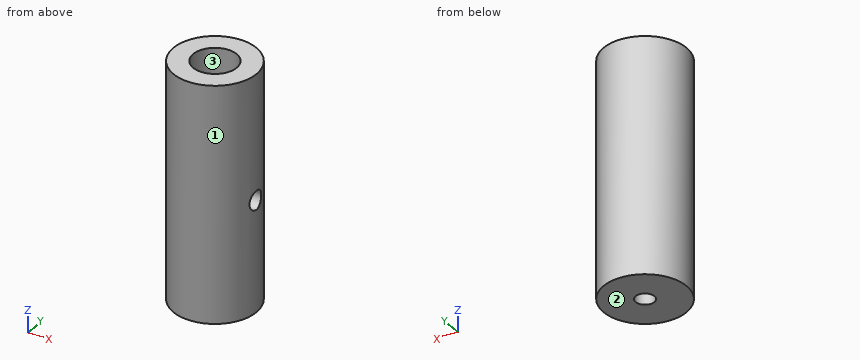
Autodesk Inventor part; units mm, degrees
ref_plane "Work Plane1" through (4.7625, 0, 0) normal (1, 0, 0) x (0, 1, 0)
ref_plane "XZ Plane" through (0, 0, 0) normal (0, 1, 0) x (-1, 0, 0)
ref_plane "XY Plane" through (0, 0, 0) normal (0, 0, 1) x (1, 0, 0)
sketch "Sketch1" plane through (0, 0, 0) normal (0, 0, 1) x (1, 0, 0)
  circle A0 centre (0, 0) radius 4.7625
  dimension "d0" = 9.525
extrude "Extrusion1" add sketch "Sketch1" along normal blind 26.9875
sketch "Sketch2" plane through (0, 0, 26.9875) normal (0, 0, 1) x (1, 0, 0)
  point P0 (0, 0)
  point P1 (0, 0)
hole "Hole1" at (0, 0, 26.9875) direction (0, 0, -1) diameter 5 depth 20.6375 tip angle 118
sketch "Sketch3" plane through (0, 0, 0) normal (0, 0, -1) x (-1, 0, 0)
  circle A0 centre (0, 0) radius 4.7625
hole "Hole2" at (0, 0, 0) direction (0, 0, 1) diameter 2.159 depth 8.8646 tip angle 118
ref_plane "Work Plane1" through (4.7625, 0, 0) normal (1, 0, 0) x (0, 1, 0)
sketch "Sketch4" plane through (4.7625, 0, 0) normal (1, 0, 0) x (0, 1, 0)
  line L0 (-2.5, 26.9875) -> (2.5, 26.9875)
  line L1 (0, 26.9875) -> (0, 12.7)
  point P0 (0, 0)
  dimension "d18" = 14.2875
hole "Hole3" at (4.7625, 0, 12.7) direction (-1, 0, 0) diameter 2.159 depth 3.81 tip angle 118
properties part number "coupler"
Verification items for the finished model (mm, model axes). Face numbers are marked on the shaded views. Give positions to 0.01 mm unless a question says otherwise; leave off trailing zeros. Write each loop counter-clockwise with the first axis right and the second up, starting at its lowest first coordinate (ties: lowest second). Pieces come first, ordered by that corner, then holes.
(1) Gauge pin test, flat end, axial feed: pin 1 (1.5 mm diameter, centred on y = 2, z = 11.5, fed in from +X). Record the tip position at first contact, or that the pin passes through.
(2) Material ranges on line 1 (Z direction, x = 2.9, y = 0); line 2 (Y direction, x = 0, z = 15.25); line 3 (Y direction, x = 1, z = 23.75), recorded low to high.
(3) Cross-section at C-C (y = 3.25). Enter the section's corners in (x, z).
(4) Mould release check, pull along Y, two halves, no side actions. Record for the marked faces 1, 2 and 3: +Y half, -Y half, draft (parallel to the pull), parting line (faces both ways), or undercut.
(5) Cross-section at A-A (x = 0). Enter the section's corners in (y, z), plus the area to 3 significant figures.
(6) Cross-section at B-B (z = 2.75). Enter the section's corners in (x, y) (1 decimal).
(7) Cross-section at D-D (z = 7.75). Enter the section's corners in (x, y) (1 decimal).
Worked out:
1. pin 1: stops at x = 4.6
2. line 1: z = 0 to 11.62, 13.78 to 26.99
2. line 2: y = -4.76 to -2.5, 2.5 to 4.76
2. line 3: y = -4.66 to -2.29, 2.29 to 4.66
3. outline: (-3.48, 0) - (3.48, 0) - (3.48, 26.99) - (-3.48, 26.99) - close
4. face 1: parting line
4. face 2: draft
4. face 3: undercut
5. outline: (-4.76, 0) - (-1.08, 0) - (-1.08, 5.5) - (-2.5, 6.35) - (-2.5, 26.99) - (-4.76, 26.99) - close; (1.08, 0) - (4.76, 0) - (4.76, 26.99) - (2.5, 26.99) - (2.5, 6.35) - (1.08, 5.5) - close
5. area: 139 mm2
6. outline: circle Ø9.5 at (0, 0); hole circle Ø2.2 at (0, 0)
7. outline: circle Ø9.5 at (0, 0); hole circle Ø5 at (0, 0)
